Design review of the part built by this model. Coordinates are the model's own, in mm. A direction names the side the tool comes from. Round coordinates to 2 decimals unless told otherwise and drop trailing zeros. Write each loop counter-clockwise with the first axis right and the second up, starting at its lowest first coordinate (ties: lowest second). Pieces come first, ordered by that corner, then holes. Notation, with made-up numbers: M 73.5,-37 L 112.5,-37 A8 cw 112.5,-24 Z; hole C 22,89.5 d5. An arc over 180 degrees is marked long. Use CSV: the item, a comma, the result in double quotes.
from build123d import *

# Parameters (mm, degrees)
ESQUISSE1_W        = 90
ESQUISSE1_H        = 45
ESQUISSE2_W        = 79.950738566
ESQUISSE2_H        = 1563.706247811
BOSS_EXTRU_1_DEPTH = 50
BOSS_EXTRU_2_DEPTH = 29
ESQUISSE5_W        = 60
ESQUISSE5_H        = 29
BOSS_EXTRU_3_DEPTH = 29
BOSS_EXTRU_4_DEPTH = 90
ESQUISSE9_W        = 128
ESQUISSE9_H        = 160.5
BOSS_EXTRU_5_DEPTH = 10


with BuildPart() as part:
    # Esquisse1 → Révolution1 (revolve)
    with BuildSketch(Plane.XY, mode=Mode.PRIVATE) as r_volution1_sk:
        with Locations((45, 22.5)):
            Rectangle(ESQUISSE1_W, ESQUISSE1_H)
    revolve(r_volution1_sk.sketch.rotate(Axis((0, 45, 0), (0, -1, 0)), 180), axis=Axis((0, 45, 0), (0, -1, 0)))

    # Esquisse2 → Boss.-Extru.1 (add)
    with BuildSketch(Plane(origin=(0, 45, 0), x_dir=(1, 0, 0), z_dir=(0, 1, 0))):
        with Locations((39.975369283, 629.271080586)):
            Rectangle(ESQUISSE2_W, ESQUISSE2_H)
    extrude(amount=BOSS_EXTRU_1_DEPTH)

    # Esquisse3 → Boss.-Extru.2 (add)
    with BuildSketch(Plane(origin=(0, 45, 0), x_dir=(1, 0, 0), z_dir=(0, 1, 0))):
        Polygon((-278.5, 30), (0, 30), (0, -30), (-278.5, -30), (-278.5, -35), (-348.5, -35), (-348.5, -30), (-348.5, 30), (-348.5, 35), (-278.5, 35), align=None)
    extrude(amount=BOSS_EXTRU_2_DEPTH)

    # Esquisse5 → Boss.-Extru.3 (add)
    with BuildSketch(Plane(origin=(79.950738566, 0, 0), x_dir=(0, 0, -1), z_dir=(1, 0, 0))):
        with Locations((0, 59.5)):
            Rectangle(ESQUISSE5_W, ESQUISSE5_H)
    extrude(amount=BOSS_EXTRU_3_DEPTH)

    # Esquisse6 → Boss.-Extru.4 (add)
    with BuildSketch(Plane(origin=(0, 74, 0), x_dir=(1, 0, 0), z_dir=(0, 1, 0))):
        Polygon((-348.5, 35), (-278.5, 35), (-278.5, -30), (-278.5, -35), (-348.5, -35), (-348.5, -30), align=None)
    extrude(amount=BOSS_EXTRU_4_DEPTH)

    # Esquisse9 → Boss.-Extru.5 (add)
    with BuildSketch(Plane(origin=(0, 164, 0), x_dir=(1, 0, 0), z_dir=(0, 1, 0))):
        with Locations((-313.5, 0)):
            Rectangle(ESQUISSE9_W, ESQUISSE9_H)
    extrude(amount=BOSS_EXTRU_5_DEPTH)


solid = part.part
1) For pin 1 Ø3 at (y, z) = (79, -272.5) entering from -X; pin 2 Ø25 at (y, z) = (66.5, -861) entering from +X; pin 3 Ø24 at (x, z) = (48, 93.5) entering from -Y, all flat-tipped, find the tip position at first contact; note any pin that passes through.
Answers:
pin 1,"x = 0"
pin 2,"x = 79.95"
pin 3,"y = 45"
2) Add section B-B on y = 109.5. Write out the cut boundary in (x, z), then the cut area to 3 significant figures.
Answers:
outline,"M -348.5,-35 L -278.5,-35 L -278.5,35 L -348.5,35 Z"
area,"4,900 mm²"
3) Add section A-A on z = 56. Write out the cut boundary in (x, y).
Answers:
outline,"M -377.5,164 L -249.5,164 L -249.5,174 L -377.5,174 Z; M -70.46,0 L 70.46,0 L 70.46,45 L 79.95,45 L 79.95,95 L 0,95 L 0,45 L -70.46,45 Z"
4) Add section D-D on z = -128. Write out the cut boundary in (x, y).
Answers:
outline,"M 0,45 L 79.95,45 L 79.95,95 L 0,95 Z"
5) Wall thickness on line 1 along X through (y, z) = (83, -1266); line 2 along Y through (x, z) = (64, 63); line 3 along Z through (x, y) = (-63, 65): over which ranges is each line inside the solid? List them lowest first. Write a range as [from, to].
Answers:
line 1,"[0, 79.95]"
line 2,"[0, 95]"
line 3,"[-30, 30]"
6) Machinability: for faces 1 (the face through (94, 59, -30)), 2 (the face through (-348.5, 104, 0)), 3 (the face through (-313, 104, 35)), which of the approach directions +Z, -Z, +X, -X, +Y, -Y give a long, thin tool a straight path to every point of the face, cutting with its end or side? Answer none if there is none.
Answers:
face 1,"-Z, +X, +Y"
face 2,"+Z, -Z, -X, -Y"
face 3,"+Z, -X, -Y"
7) Add section C-C on x = -50.5. Write out the cut boundary in (y, z), then the cut area to 3 significant figures.
Answers:
outline,"M 0,-74.5 L 45,-74.5 L 45,-30 L 74,-30 L 74,30 L 45,30 L 45,74.5 L 0,74.5 Z"
area,"8,440 mm²"
8) The part is to be moulded in two halves that separate along X. For faces 4 (the face through (-137, 74, 0)), 5 (the face through (108.951, 60, 0)), 6 (the face through (-137, 59, 30)), 7 (the face through (94, 74, 0)), say which applies: released by +X, released by -X, zero draft, split by the parting line, or undercut.
Answers:
face 4,"undercut"
face 5,"released by +X"
face 6,"undercut"
face 7,"zero draft"
